Here's how the part is built. I have some questions about the finished solid (model axes, mm). Face numbers are marked on the shaded views. A direction names the side the tool comes from. Give positions to 0.01 mm unless a question says otherwise; leave off trailing zeros. Loops run counter-clockwise (first coordinate to the right, second up) from the corner with the lowest first, then second, coordinate; pieces in that order, holes last. Notation, with made-up numbers: M 17.5,-30.5 L 60.5,-30.5 A15 cw 60.5,-3.5 Z; hole C -30.75,22.5 d6. An arc over 180 degrees is marked long. Answer as CSV lines item,"result". Start each with the question number.
Item 1: I want a section at C-C on x = -2.5. List the corners of the cut face in (y, z) for me, plus the area to 3 significant figures.
Item 2: If we mould it in two halves opening along X, with no side actions, what happens to the marked faces 5, 6 and 7? For each: released by +X, released by -X, zero draft, split by the parting line, or undercut.
Item 3: I want a section at A-A on y = 15. List the corners of the cut face in (x, z) for me.
Item 4: Will these pins go through, and if not, where does the flat tip stop? P1, Ø5, axis at x = -17.5, z = -17.5, coming from the +Y side; P2, Ø3, axis at x = -4, z = -31.5, coming from the +Y side; P3, Ø10, axis at x = -2, z = 16.5, coming from the -Y side.
Item 5: If I drill on line 1 along X through (y, z) = (33, -17.5); line 2 along Z through (x, y) = (-17.5, 36); line 3 along X through (y, z) = (10.5, 5), over which ranges is the centre line in solid material (lowest first)? Write a range as from..to.
Item 6: I want a section at D-D on y = 37. List the corners of the cut face in (x, z) for me.
Item 7: For the marked faces 1, 2, 3 and 4, which set-ups out of +Z, -Z, +X, -X, +Y, -Y let a thin tool reach every point of the face, with its end or its side?
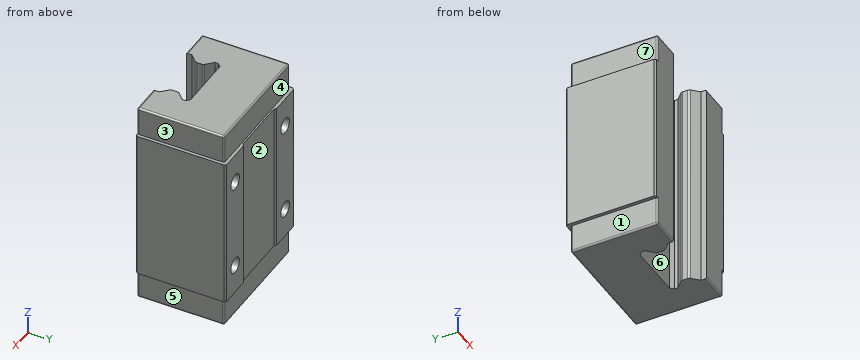
from build123d import *

# Parameters (mm, degrees)
SKETCH1_W           = 48
SKETCH1_H           = 34.2
BOSS_EXTRUDE1_DEPTH = 28.75
SKETCH2_W           = 45.5
SKETCH2_H           = 32.95
BOSS_EXTRUDE2_DEPTH = 39.6
SKETCH3_W           = 23
SKETCH3_H           = 19.2
CUT_EXTRUDE1_DEPTH  = 92.916483832
BOSS_EXTRUDE3_DEPTH = 79.2
CHAMFER1_SIZE       = 1.25
FILLET1_R           = 1.25
SKETCH5_W           = 23
SKETCH5_H           = 0.62
CUT_EXTRUDE2_DEPTH  = 83.750966762
CHAMFER2_SIZE       = 0.62
FILLET2_R           = 0.62
SKETCH6_R           = 3
CUT_EXTRUDE3_DEPTH  = 9


with BuildPart() as part:
    # Sketch1 → Boss-Extrude1 (new, symmetric)
    with BuildSketch(Plane.XY):
        with Locations((0, 22.9)):
            Rectangle(SKETCH1_W, SKETCH1_H)
    extrude(amount=BOSS_EXTRUDE1_DEPTH, both=True)

    # Sketch2 → Boss-Extrude2 (add, symmetric)
    with BuildSketch(Plane.XY):
        with Locations((0, 22.275)):
            Rectangle(SKETCH2_W, SKETCH2_H)
    extrude(amount=BOSS_EXTRUDE2_DEPTH, both=True)

    # Sketch3 → Cut-Extrude1 (cut, through all)
    with BuildSketch(Plane.XY.offset(39.6)):
        with Locations((0, 9.6)):
            Rectangle(SKETCH3_W, SKETCH3_H)
    extrude(amount=-CUT_EXTRUDE1_DEPTH, mode=Mode.SUBTRACT)

    # Sketch4 → Boss-Extrude3 (add)
    with BuildSketch(Plane.XY.offset(39.6)):
        Polygon((-11.5, 16.7), (-11.5, 7.95), (-8.583333333, 10.866666667), (-8.583333333, 13.783333333), align=None)
        Polygon((8.583333333, 13.783333333), (11.5, 16.7), (11.5, 7.95), (8.583333333, 10.866666667), align=None)
    extrude(amount=-BOSS_EXTRUDE3_DEPTH)

    # Chamfer1
    chamfer1_edges = [part.edges().sort_by_distance(p)[0] for p in [
        (11.5, 19.2, 0),
        (-11.5, 19.2, 0),
    ]]
    chamfer(chamfer1_edges, length=CHAMFER1_SIZE)

    # Fillet1
    fillet1_edges = [part.edges().sort_by_distance(p)[0] for p in [
        (-8.583333333, 10.866666667, 0),
        (-8.583333333, 13.783333333, 0),
        (8.583333333, 13.783333333, 0),
        (8.583333333, 10.866666667, 0),
    ]]
    fillet(fillet1_edges, radius=FILLET1_R)

    # Sketch5 → Cut-Extrude2 (cut, through all)
    with BuildSketch(Plane.XY.offset(28.75)):
        with Locations((0, 39.69)):
            Rectangle(SKETCH5_W, SKETCH5_H)
    extrude(amount=-CUT_EXTRUDE2_DEPTH, mode=Mode.SUBTRACT)

    # Chamfer2
    chamfer2_edges = [part.edges().sort_by_distance(p)[0] for p in [
        (-11.5, 39.38, 0),
        (11.5, 39.38, 0),
        (24, 5.8, 0),
        (-24, 5.8, 0),
        (-24, 40, 0),
        (24, 40, 0),
    ]]
    chamfer(chamfer2_edges, length=CHAMFER2_SIZE - 0.0001)  # a hair under: the kernel refuses the full size

    # Fillet2
    fillet2_edges = [part.edges().sort_by_distance(p)[0] for p in [
        (-22.75, 38.75, 34.175),
        (-22.75, 5.8, 34.175),
        (22.75, 5.8, 34.175),
        (22.75, 38.75, 34.175),
        (-22.75, 38.75, -34.175),
        (-22.75, 22.275, -39.6),
        (-22.75, 5.8, -34.175),
        (-17.125, 5.8, -39.6),
        (22.75, 5.8, -34.175),
        (22.75, 22.275, -39.6),
        (22.75, 38.75, -34.175),
        (0, 38.75, -39.6),
        (-22.75, 22.275, 39.6),
        (-17.125, 5.8, 39.6),
        (22.75, 22.275, 39.6),
        (0, 38.75, 39.6),
        (17.125, 5.8, 39.6),
        (17.125, 5.8, -39.6),
    ]]
    fillet(fillet2_edges, radius=FILLET2_R)

    # Sketch6 → Cut-Extrude3 (cut)
    with BuildSketch(Plane(origin=(0, 40, 0), x_dir=(1, 0, 0), z_dir=(0, 1, 0))):
        with Locations(Location((-17.5, -17.5, 0), (0, 0, 180))):
            Circle(SKETCH6_R)
        with Locations(Location((17.5, -17.5, 0), (0, 0, 180))):
            Circle(SKETCH6_R)
    cut_extrude3 = extrude(amount=-CUT_EXTRUDE3_DEPTH, mode=Mode.SUBTRACT)

    # Mirror1: Cut-Extrude3 across plane
    add(cut_extrude3.mirror(Plane.XY), mode=Mode.SUBTRACT)


solid = part.part
Result:
1,outline,"M 19.2,-39.6 L 38.13,-39.6 A0.62 ccw 38.75,-38.98 L 38.75,-28.75 L 39.38,-28.75 L 39.38,28.75 L 38.75,28.75 L 38.75,38.98 A0.62 ccw 38.13,39.6 L 19.2,39.6 Z"
1,area,"1,580 mm^2"
2,face 5,"released by +X"
2,face 6,"undercut"
2,face 7,"released by -X"
3,outline,"M -24,-28.75 L -22.75,-28.75 L -22.75,-38.98 A0.62 ccw -22.13,-39.6 L -9.8,-39.6 L -9.8,39.6 L -22.13,39.6 A0.62 ccw -22.75,38.98 L -22.75,28.75 L -24,28.75 Z; M 9.8,-39.6 L 22.13,-39.6 A0.62 ccw 22.75,-38.98 L 22.75,-28.75 L 24,-28.75 L 24,28.75 L 22.75,28.75 L 22.75,38.98 A0.62 ccw 22.13,39.6 L 9.8,39.6 Z"
4,P1,"y = 31"
4,P2,"y = 38.75"
4,P3,"y = 19.2"
5,line 1,"-24..-20.5, -14.5..14.5, 20.5..24"
5,line 2,"-39.6..-20.5, -14.5..14.5, 20.5..39.6"
5,line 3,"-24..-8.95, 8.95..24"
6,outline,"M -24,-28.75 L -22.75,-28.75 L -22.75,-38.98 A0.62 ccw -22.13,-39.6 L 22.13,-39.6 A0.62 ccw 22.75,-38.98 L 22.75,-28.75 L 24,-28.75 L 24,28.75 L 22.75,28.75 L 22.75,38.98 A0.62 ccw 22.13,39.6 L -22.13,39.6 A0.62 ccw -22.75,38.98 L -22.75,28.75 L -24,28.75 Z; hole C -17.5,-17.5 d6; hole C -17.5,17.5 d6; hole C 17.5,-17.5 d6; hole C 17.5,17.5 d6"
7,face 1,"-Z, -X, +Y, -Y"
7,face 2,"+Z, -Z, +Y"
7,face 3,"+Z, +X, +Y, -Y"
7,face 4,"+Z, +X, -X, +Y"
